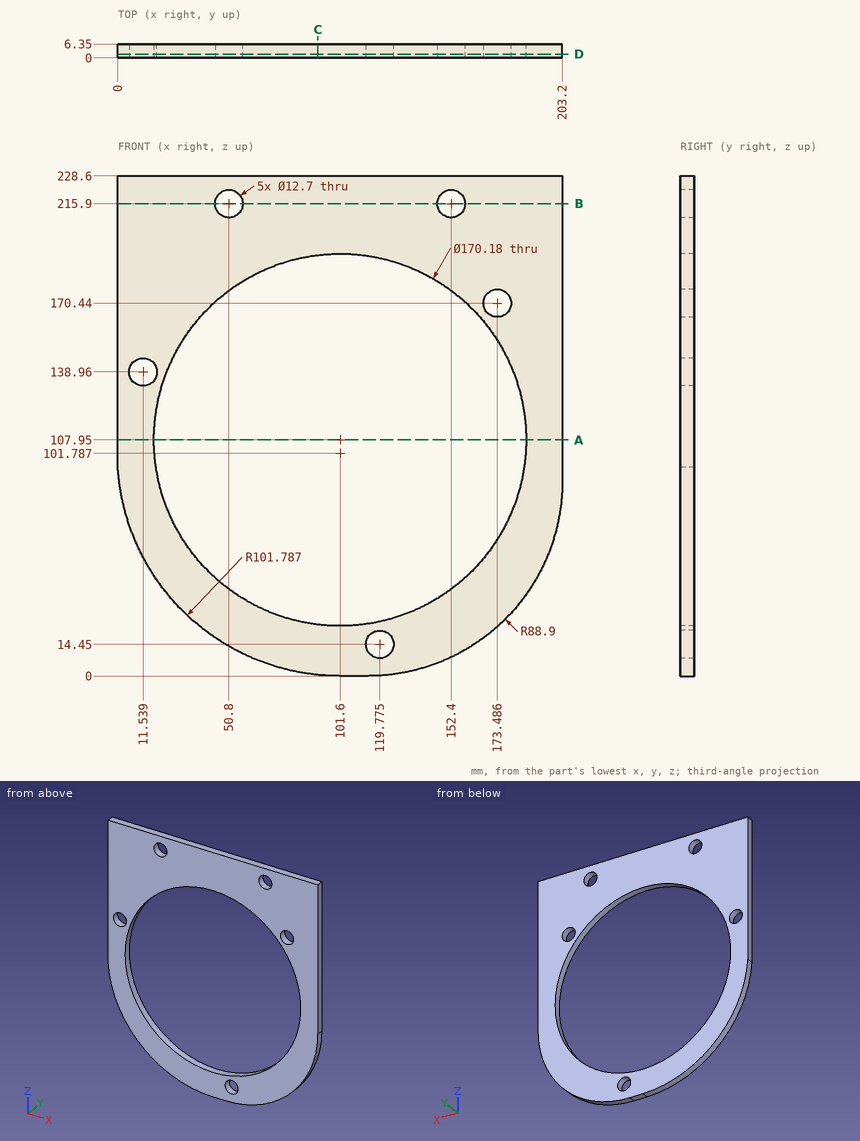
Source: three-view drawing plus pictorial views. Frame: mm from the lowest corner of the part. Round coordinates to 2 decimals unless told otherwise and drop trailing zeros. Write each loop counter-clockwise with the first axis right and the second up, starting at its lowest first coordinate (ties: lowest second). Pieces come first, ordered by that corner, then holes. Notation, with made-up numbers: M 8.25,40.5 L 18.25,40.5 A11 ccw 18.25,57.5 Z; hole C 72,28.5 d7. An arc over 180 degrees is marked long. Write item = value, one per line.
Item 1: Material intervals for line 1 along X through (y, z) = (3, 215.9); line 2 along Z through (x, y) = (152.4, 1.5); line 3 along X through (y, z) = (5.25, 171.5) (1 decimal), sorted ascending. Write a range as [from, to].
Findings:
line_1 = [0, 44.45], [57.15, 146.05], [158.75, 203.2]
line_2 = [8.58, 39.69], [176.21, 209.55], [222.25, 228.6]
line_3 = [0, 45], [158.2, 167.2], [179.7, 203.2]
Item 2: Section query A-A on z = 107.95. Return loops of the section in (x, y), then the cut area to 3 significant figures.
Findings:
outline = M 0,0 L 16.51,0 L 16.51,6.35 L 0,6.35 Z; M 186.69,0 L 203.2,0 L 203.2,6.35 L 186.69,6.35 Z
area = 210 mm^2
Item 3: Section query B-B on z = 215.9. Return loops of the section in (x, y).
Findings:
outline = M 0,0 L 44.45,0 L 44.45,6.35 L 0,6.35 Z; M 57.15,0 L 146.05,0 L 146.05,6.35 L 57.15,6.35 Z; M 158.75,0 L 203.2,0 L 203.2,6.35 L 158.75,6.35 Z
Item 4: Section query C-C on x = 91.5. Return loops of the section in (y, z).
Findings:
outline = M 0,0.5 L 6.35,0.5 L 6.35,23.46 L 0,23.46 Z; M 0,192.44 L 6.35,192.44 L 6.35,228.6 L 0,228.6 Z
Item 5: Section query D-D on y = 1.75. State how many separate pieces and enclosed holes the cut face has, then the cut area to 3 significant figures.
Findings:
separate_pieces = 1
enclosed_holes = 6
area = 19,200 mm^2
